Could you check a few things on this model? Use its own coordinates, in mm. A direction names the side the tool comes from. Coordinates: 2 decimals unless noted, no trailing zeros. Loops run counter-clockwise (first coordinate to the right, second up) from the corner with the lowest first, then second, coordinate; pieces in that order, holes last. Notation, with made-up numbers: (65.5, 1.5) -> (77.5, 1.5) arc R3 ccw to (77.5, 5.5) -> close; hole circle Ø8 at (-26, 1.25). An arc over 180 degrees is marked (long way). One line per question, with ' | ' between items. Start each with the question number.
(1) If we mould it in two halves opening along Z, with no side actions, what happens to faces 3 (the face through (-29.39, 6.06, -29.1)), 4 (the face through (-7, 0, 0)), 5 (the face through (3.584, 6.064, -2.285))? For each: pulls with the +Z half, pulls with the -Z half, needs draft (parallel to the pull), parting line crosses it, or undercut.
(2) I'm going to push flat-ended pins straight in: pin 1 Ø8 at (x, z) = (-14.99, 15.33) entering from +Y; pin 2 Ø6.5 at (x, z) = (-17.5, 16.5) entering from +Y. Where does each tip first touch, or does it pass through?
(3) Which directions (+Z, -Z, +X, -X, +Y, -Y) give clear straight access to the entire face, cutting with the end or side of a thin tool? Please do faces 1 (the face through (17, 3.9, 20)), 2 (the face through (11.014, 1.923, -12.593)).
(4) Suppose I cut it at D-D (x = -16.5). Please give me the cut outline in (y, z).
(5) Suppose I cut it at C-C (z = 0). Please give me the cut outline in (x, y), plus the area to 3 significant figures.
(6) Suppose I cut it at A-A (x = 0). Please give me the cut outline in (y, z), plus the area to 3 significant figures.
(7) If I drill on line 1 along Z through (x, y) = (12, 5.25); line 2 along X through (y, z) = (8, -17); line 3 along Z through (x, y) = (9, 7), over which ranges is the centre line in solid material (lowest first)?
(8) Suppose I cut it at B-B (z = 14). Please give me the cut outline in (x, y), plus the area to 3 significant figures.
```python
from build123d import *

# Parameters (mm, degrees)
SKETCH_1_R              = 4.5
EXTRUDE_1_DEPTH         = 12.3
HOLE_WIZARD_M10_1_D     = 8.5
HOLE_WIZARD_M10_1_DEPTH = 24.5
HOLE_WIZARD_M10_1_TIP   = 2.553657631
SKETCH_5_R              = 6.5
CUT_EXTRUDE_1_DEPTH     = 8.4


with BuildPart() as part:
    # 草图1 → 凸台-拉伸1 (new body)
    with BuildSketch(Plane(origin=(0, 0, 0), x_dir=(1, 0, 0), z_dir=(0, 1, 0))):
        with BuildLine():
            Line((-27.993607343, -30.330536434), (28.006392657, -30.330536434))
            ThreePointArc((28.006392657, -30.330536434), (29.42060622, -29.744749996), (30.006392657, -28.330536434))
            Line((30.006392657, -28.330536434), (30.006392657, 27.669463566))
            ThreePointArc((30.006392657, 27.669463566), (29.42060622, 29.083677128), (28.006392657, 29.669463566))
            Line((28.006392657, 29.669463566), (-27.993607343, 29.669463566))
            ThreePointArc((-27.993607343, 29.669463566), (-29.407820905, 29.083677128), (-29.993607343, 27.669463566))
            Line((-29.993607343, 27.669463566), (-29.993607343, -28.330536434))
            ThreePointArc((-29.993607343, -28.330536434), (-29.407820905, -29.744749996), (-27.993607343, -30.330536434))
        make_face()
        with Locations(Location((15.006392657, -15.330536434, 0), (0, 0, 270))):
            Circle(SKETCH_1_R, mode=Mode.SUBTRACT)
        with Locations(Location((15.006392657, 14.669463566, 0), (0, 0, 270))):
            Circle(SKETCH_1_R, mode=Mode.SUBTRACT)
        with Locations(Location((-14.993607343, 14.669463566, 0), (0, 0, 270))):
            Circle(SKETCH_1_R, mode=Mode.SUBTRACT)
        with Locations(Location((-14.993607343, -15.330536434, 0), (0, 0, 270))):
            Circle(SKETCH_1_R, mode=Mode.SUBTRACT)
    extrude(amount=EXTRUDE_1_DEPTH)

    # M10 螺纹孔1
    with Locations(Plane.ZX.offset(12.3)):
        with Locations((0, 0)):
            Hole(HOLE_WIZARD_M10_1_D / 2, depth=HOLE_WIZARD_M10_1_DEPTH)
            with Locations((0, 0, -(HOLE_WIZARD_M10_1_DEPTH + HOLE_WIZARD_M10_1_TIP / 2))):  # 118° drill point
                Cone(0, HOLE_WIZARD_M10_1_D / 2, HOLE_WIZARD_M10_1_TIP, mode=Mode.SUBTRACT)

    # 草图5 → 切除-拉伸1 (cut)
    with BuildSketch(Plane(origin=(0, 12.3, 0), x_dir=(1, 0, 0), z_dir=(0, 1, 0))):
        with Locations(Location((-14.993607343, 14.669463566, 0), (0, 0, 270))):
            Circle(SKETCH_5_R)
        with Locations(Location((15.006392657, 14.669463566, 0), (0, 0, 270))):
            Circle(SKETCH_5_R)
        with Locations(Location((15.006392657, -15.330536434, 0), (0, 0, 270))):
            Circle(SKETCH_5_R)
        with Locations(Location((-14.993607343, -15.330536434, 0), (0, 0, 270))):
            Circle(SKETCH_5_R)
    extrude(amount=-CUT_EXTRUDE_1_DEPTH, mode=Mode.SUBTRACT)


solid = part.part
```
Checks:
1) face 3: pulls with the -Z half | face 4: needs draft | face 5: undercut
2) pin 1: passes through | pin 2: stops at y = 3.9
3) face 1: +Y | face 2: +Y, -Y
4) outline: (0, -29.67) -> (12.3, -29.67) -> (12.3, -20.99) -> (3.9, -20.99) -> (3.9, -18.91) -> (0, -18.91) -> close; (0, -10.43) -> (3.9, -10.43) -> (3.9, -8.35) -> (12.3, -8.35) -> (12.3, 9.01) -> (3.9, 9.01) -> (3.9, 11.09) -> (0, 11.09) -> close; (0, 19.57) -> (3.9, 19.57) -> (3.9, 21.65) -> (12.3, 21.65) -> (12.3, 30.33) -> (0, 30.33) -> close
5) outline: (-29.99, 0) -> (-4.25, 0) -> (-4.25, 12.3) -> (-29.99, 12.3) -> close; (4.25, 0) -> (30.01, 0) -> (30.01, 12.3) -> (4.25, 12.3) -> close | area: 633 mm^2
6) outline: (0, -29.67) -> (12.3, -29.67) -> (12.3, -4.25) -> (0, -4.25) -> close; (0, 4.25) -> (12.3, 4.25) -> (12.3, 30.33) -> (0, 30.33) -> close | area: 633 mm^2
7) line 1: z = -29.67 to -20.43, -8.91 to 9.57, 21.09 to 30.33 | line 2: x = -29.99 to -21.06, -8.93 to 8.94, 21.07 to 30.01 | line 3: z = -29.67 to -17.15, -12.18 to 12.85, 17.82 to 30.33
8) outline: (-29.99, 0) -> (-19.29, 0) -> (-19.29, 3.9) -> (-21.36, 3.9) -> (-21.36, 12.3) -> (-29.99, 12.3) -> close; (-10.69, 0) -> (10.71, 0) -> (10.71, 3.9) -> (8.64, 3.9) -> (8.64, 12.3) -> (-8.63, 12.3) -> (-8.63, 3.9) -> (-10.69, 3.9) -> close; (19.31, 0) -> (30.01, 0) -> (30.01, 12.3) -> (21.37, 12.3) -> (21.37, 3.9) -> (19.31, 3.9) -> close | area: 457 mm^2
